Autodesk Inventor part; units mm, degrees
ref_plane "YZ Plane" through (0, 0, 0) normal (1, 0, 0) x (0, 1, 0)
ref_plane "XZ Plane" through (0, 0, 0) normal (0, 1, 0) x (-1, 0, 0)
ref_plane "XY Plane" through (0, 0, 0) normal (0, 0, 1) x (1, 0, 0)
sketch "Sketch1" plane through (0, 0, 0) normal (0, 0, 1) x (1, 0, 0)
  line L0 (-12.8542, 0) -> (25.2458, 0)
  line L1 (25.2458, 0) -> (25.2458, 50.8)
  line L2 (25.2458, 50.8) -> (-12.8542, 50.8)
  line L3 (-12.8542, 50.8) -> (-12.8542, 0)
  circle A0 centre (-4.5992, 21.2852) radius 3.175
  line L4 (-7.7742, 21.2852) -> (-7.7742, 0)
  line L5 (-1.9984, 23.1063) -> (14.1808, 0)
  line L6 (-5.8785, 50.8) -> (25.2458, 6.35)
  point P0 (0, 0)
  dimension "d0" = 38.1
  dimension "d1" = 50.8
  dimension "d2" = 6.35
  dimension "d3" = 8.255
  dimension "d4" = 21.2852
  dimension "d5" = 6.35
  dimension "d6" = 35
extrude "Extrusion1" add sketch "Sketch1" along normal blind 12.7 contours L3 L2 L6 L1 L0 L5 A0 L4
sketch "Sketch2" plane through (-5.8785, 50.8, 12.7) normal (0.8192, 0.5736, 0) x (0, 0, -1)
  circle A0 centre (6.35, -8.5344) radius 2.8702
  circle A1 centre (6.35, -18.6944) radius 2.8702
  circle A2 centre (6.35, -30.1244) radius 2.8702
  circle A3 centre (6.35, -44.0944) radius 2.8702
  line L0 (12.7, 0) -> (0, 0)
  line L1 (12.7, -54.2634) -> (12.7, 0)
  point P0 (12.7, -44.9847)
  dimension "d9" = 5.7404
  dimension "d10" = 5.7404
  dimension "d11" = 5.7404
  dimension "d12" = 5.7404
  dimension "d13" = 8.5344
  dimension "d14" = 6.35
  dimension "d16" = 30.1244
  dimension "d17" = 44.0944
  dimension "d18" = 18.6944
extrude "Extrusion2" cut sketch "Sketch2" against normal blind 10.16
sketch "Sketch3" plane through (-12.8542, 0, 0) normal (-1, 0, 0) x (0, 0, 1)
  line L0 (0, 50.8) -> (0, 0)
  line L1 (0, 0) -> (12.7, 0)
  point P0 (6.35, 46.99)
  point P1 (6.35, 3.81)
  dimension "d21" = 6.35
  dimension "d22" = 6.35
  dimension "d23" = 46.99
  dimension "d24" = 3.81
hole "Hole1" at (-12.8542, 46.99, 6.35) at (-12.8542, 3.81, 6.35) direction (1, 0, 0) diameter 3.302 depth 7.62 tip angle 118
equation "\"d10\" = d9"
equation "\"d11\" = d9"
equation "\"d12\" = d9"
properties part number "Punch Holder" material "Stainless Steel"
Geometry: final body of the model. Coordinates: model frame, mm. A direction names the side the tool comes from. Coordinates: 2 decimals unless noted, no trailing zeros. Order: outer loops, then holes, each group sorted by start corner. A loop starts at its lowest first (then second) coordinate and runs counter-clockwise, first axis right, second up. Notation, with made-up numbers: M 38.5,15 L 90.5,15 A22 ccw 90.5,29 Z; hole C 81.25,85.25 d7. An arc over 180 degrees is marked long. Answer in a Markdown table with one row per item. Add a question column.
Q1. Line query: L1, parallel to Z at x = -9.75, y = 46.99; L2, parallel to Y at x = -10, z = 6.35; L3, parallel to Y at x = -10.5, z = 6.35. Output: solid intervals per line, ascending.
Q2. Contact query for flat-ended pins moving along their axis: P1, Ø2, axis at y = 27.5, z = 4.5, coming from the +X side; P2, Ø2, axis at x = 16.5, z = 4.5, coming from the +Y side; P3, Ø2, axis at x = 7, z = 9, coming from the +Y side. Output: stop coordinate, or through.
Q3. Reachability of faces 4 (the flat face through (9.466, 28.886, 6.261)), 5 (the flat face through (-7.774, 11, 6)), 6 (the flat face through (11.07, 8.88, 6.39)) from +Z, -Z, +X, -X, +Y, -Y: full face, straight path, thin tool, end or side. Return the list, or none.
Q4. Section query C-C on x = 23. Return the cut outline in (y, z).
Q5. Mould query, pull axis Y, two halves, no side actions, for faces 1 (the flat face through (20, 0, 6)), 2 (the cylindrical face through (-8.99, 48.6, 5.99)), 3 (the flat face through (25.246, 3, 6)). Classes: released by +Y, released by -Y, zero draft, split by the parting line, or undercut.
Q6. Section query A-A on y = 3.81. Return the cut outline in (x, z), and give its area (3 significant figures).
Completed:
| question | item | result |
|---|---|---|
| 1 | L1 | z = 0 to 4.7, 8 to 12.7 |
| 1 | L2 | y = 0 to 2.16, 5.46 to 38.97, 41 to 45.34, 48.64 to 50.8 |
| 1 | L3 | y = 0 to 2.16, 5.46 to 39.68, 40.65 to 45.34, 48.64 to 50.8 |
| 2 | P1 | stops at x = 10.82 |
| 2 | P2 | stops at y = 20.27 |
| 2 | P3 | stops at y = 33.84 |
| 3 | face 4 | +Z, -Z, +X, +Y |
| 3 | face 5 | +Z, -Z, -Y |
| 3 | face 6 | none |
| 4 | outline | M 0,0 L 9.56,0 L 9.56,12.7 L 0,12.7 Z |
| 5 | face 1 | released by -Y |
| 5 | face 2 | undercut |
| 5 | face 3 | zero draft |
| 6 | outline | M -12.85,0 L -7.77,0 L -7.77,4.7 L -12.85,4.7 Z; M -12.85,8 L -7.77,8 L -7.77,12.7 L -12.85,12.7 Z; M 11.51,0 L 25.25,0 L 25.25,12.7 L 11.51,12.7 Z |
| 6 | area | 222 mm2 |
